Can you work these out from the model? Positions are in its coordinate system, mm. Round coordinates to 2 decimals unless told otherwise and drop trailing zeros. Order: outer loops, then holes, each group sorted by start corner. A loop starts at its lowest first (then second) coordinate and runs counter-clockwise, first axis right, second up.
Q1. If I drill on line 1 (X direction, y = 6, z = -21.5); line 2 (Z direction, x = 21, y = -2); line 3 (Y direction, x = -2, z = -38.1) (3 decimals), over which ranges is the centre line in solid material (lowest first)?
Q2. If we section it at B-B (y = 22.5): Please give me the cut outline in (x, z).
Q3. If we section it at C-C (z = -38.1): Please give me the cut outline in (x, y) (3 decimals), plus the area to 3 significant figures.
Q4. If we section it at D-D (z = -26): Please give me the cut outline in (x, y).
Q5. Will this pin go through, and if not, where does the flat tip stop? P1, Ø17, axis at y = 0, z = -38.1, coming from the -X side.
Q6. If we section it at A-A (x = 28): Please give me the cut outline in (y, z), plus the area to 3 significant figures.
from build123d import *

# Parameters (mm, degrees)
F0_W     = 63.5
F0_H     = 101.6
F1_DEPTH = 50.8
F2_T     = -2.54
F3_W     = 63.5
F3_H     = 101.6
F4_DEPTH = 2.794
F7_DEPTH = 25.4
F8_DEPTH = 25.4


with BuildPart() as f1:
    # F0 (on Right) → F1 (new body)
    with BuildSketch(Plane.YZ):
        Rectangle(F0_W, F0_H)
    extrude(amount=F1_DEPTH)

    # F2
    f2_openings = [f1.faces().sort_by_distance(p)[0] for p in [
        (0, 0, 0),
    ]]
    offset(amount=F2_T, openings=f2_openings)

    # F3 (on Right) → F4 (join)
    with BuildSketch(Plane.YZ):
        Rectangle(F3_W, F3_H)
    extrude(amount=-F4_DEPTH)

    # F5 (on face) → F7 (cut)
    with BuildSketch(Plane(origin=(-2.794, 0, 0), x_dir=(0, -1, 0), z_dir=(-1, 0, 0))):
        with BuildLine():
            ThreePointArc((6.35, 38.1), (-4.4901280605, 42.5901280605), (0, 31.75))
            ThreePointArc((0, 31.75), (4.4901280605, 33.6098719395), (6.35, 38.1))
        make_face()
        with BuildLine():
            ThreePointArc((9.525, -38.1), (6.7351920908, -31.3648079092), (0, -28.575))
            ThreePointArc((0, -28.575), (-6.7351920908, -44.8351920908), (9.525, -38.1))
        make_face()
    extrude(amount=-F7_DEPTH, mode=Mode.SUBTRACT)

    # F6 (on face) → F8 (cut)
    with BuildSketch(Plane(origin=(-2.794, 0, 0), x_dir=(0, -1, 0), z_dir=(-1, 0, 0))):
        Polygon((0, 23.1647733599), (-3.5581812263, 23.1647733599), (-3.5581812263, -27.3652244359), (0, -27.3652244359), (0, 0), align=None)
        Polygon((3.5581812263, 23.1647733599), (0, 23.1647733599), (0, 0), (0, -27.3652244359), (3.5581812263, -27.3652244359), align=None)
    extrude(amount=-F8_DEPTH, mode=Mode.SUBTRACT)


solid = f1.part
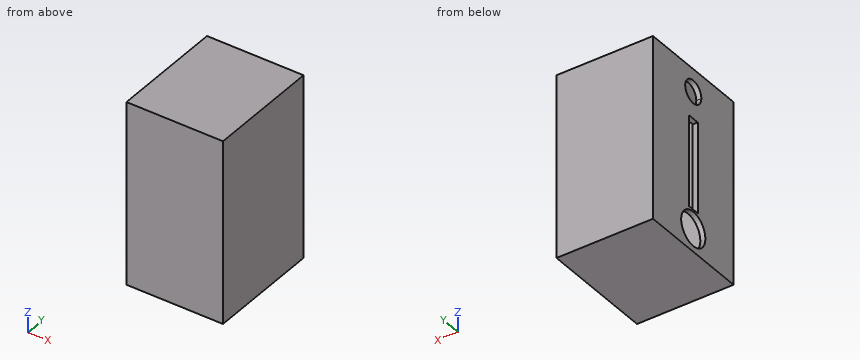
Solution:
1. line 1: x = -2.79 to 0, 48.26 to 50.8
1. line 2: z = -50.8 to -48.26, 48.26 to 50.8
1. line 3: y = -31.75 to -9.525, 9.525 to 31.75
2. outline: (-2.79, -50.8) - (50.8, -50.8) - (50.8, 50.8) - (-2.79, 50.8) - close; hole (0, -48.26) - (48.26, -48.26) - (48.26, 48.26) - (0, 48.26) - close
3. outline: (-2.794, -31.75) - (50.8, -31.75) - (50.8, 31.75) - (-2.794, 31.75) - (-2.794, 9.525) - (0, 9.525) - (0, 29.21) - (48.26, 29.21) - (48.26, -29.21) - (0, -29.21) - (0, -9.525) - (-2.794, -9.525) - close
3. area: 531 mm2
4. outline: (-2.79, -31.75) - (50.8, -31.75) - (50.8, 31.75) - (-2.79, 31.75) - (-2.79, 3.56) - (0, 3.56) - (0, 29.21) - (48.26, 29.21) - (48.26, -29.21) - (0, -29.21) - (0, -3.56) - (-2.79, -3.56) - close
5. P1: stops at x = 48.26
6. outline: (-31.75, -50.8) - (31.75, -50.8) - (31.75, 50.8) - (-31.75, 50.8) - close; hole (-29.21, -48.26) - (29.21, -48.26) - (29.21, 48.26) - (-29.21, 48.26) - close
6. area: 813 mm2
